For this review, take the finished solid that the model builds, in its own axes (mm). A direction names the side the tool comes from. Coordinates: 2 decimals unless noted, no trailing zeros. Order: outer loops, then holes, each group sorted by start corner. A loop starts at its lowest first (then second) coordinate and runs counter-clockwise, first axis right, second up.
from build123d import *

# Parameters (mm, degrees)
F1_DEPTH  = 8
F0_R      = 3.1
F0_R_2    = 1.375
F2_DEPTH  = 3
F3_DEPTH  = 8
F4_W      = 7.5
F4_H      = 5
F5_DEPTH  = 3
F4_W_2    = 15
F4_W_3    = 6
F6_DEPTH  = 3
F7_W      = 15.9
F7_H      = 5
F7_W_2    = 13.1
F8_DEPTH  = 3
F9_W      = 14.6
F9_H      = 5
F10_DEPTH = 3
F11_DEPTH = 10


with BuildPart() as f1:
    # F0 (on Top) → F1 (new body)
    with BuildSketch(Plane.XY):
        with BuildLine():
            Line((82, 59), (3, 59))
            ThreePointArc((3, 59), (-1.242641, 57.242641), (-3, 53))
            Line((-3, 53), (-3, 3))
            ThreePointArc((-3, 3), (-1.242641, -1.242641), (3, -3))
            Line((3, -3), (82, -3))
            ThreePointArc((82, -3), (86.242641, -1.242641), (88, 3))
            Line((88, 3), (88, 53))
            ThreePointArc((88, 53), (86.242641, 57.242641), (82, 59))
        make_face()
        with BuildLine():
            Line((82, 0), (3, 0))
            ThreePointArc((3, 0), (0.87868, 0.87868), (0, 3))
            Line((0, 3), (0, 53))
            ThreePointArc((0, 53), (0.87868, 55.12132), (3, 56))
            Line((3, 56), (82, 56))
            ThreePointArc((82, 56), (84.12132, 55.12132), (85, 53))
            Line((85, 53), (85, 3))
            ThreePointArc((85, 3), (84.12132, 0.87868), (82, 0))
        make_face(mode=Mode.SUBTRACT)
    extrude(amount=F1_DEPTH)

    # F0 (on Top) → F2 (join)
    with BuildSketch(Plane.XY):
        with BuildLine():
            Line((82, 59), (3, 59))
            ThreePointArc((3, 59), (-1.242641, 57.242641), (-3, 53))
            Line((-3, 53), (-3, 3))
            ThreePointArc((-3, 3), (-1.242641, -1.242641), (3, -3))
            Line((3, -3), (82, -3))
            ThreePointArc((82, -3), (86.242641, -1.242641), (88, 3))
            Line((88, 3), (88, 53))
            ThreePointArc((88, 53), (86.242641, 57.242641), (82, 59))
        make_face()
        with BuildLine():
            Line((82, 0), (3, 0))
            ThreePointArc((3, 0), (0.87868, 0.87868), (0, 3))
            Line((0, 3), (0, 53))
            ThreePointArc((0, 53), (0.87868, 55.12132), (3, 56))
            Line((3, 56), (82, 56))
            ThreePointArc((82, 56), (84.12132, 55.12132), (85, 53))
            Line((85, 53), (85, 3))
            ThreePointArc((85, 3), (84.12132, 0.87868), (82, 0))
        make_face(mode=Mode.SUBTRACT)
        with BuildLine():
            ThreePointArc((0, 3), (0.87868, 0.87868), (3, 0))
            Line((3, 0), (82, 0))
            ThreePointArc((82, 0), (84.12132, 0.87868), (85, 3))
            Line((85, 3), (85, 53))
            ThreePointArc((85, 53), (84.12132, 55.12132), (82, 56))
            Line((82, 56), (3, 56))
            ThreePointArc((3, 56), (0.87868, 55.12132), (0, 53))
            Line((0, 53), (0, 3))
        make_face()
        with Locations((3.5, 3.5)):
            Circle(F0_R, mode=Mode.SUBTRACT)
        with Locations((61.5, 3.5)):
            Circle(F0_R, mode=Mode.SUBTRACT)
        with Locations((3.5, 52.5)):
            Circle(F0_R, mode=Mode.SUBTRACT)
        with Locations((61.5, 52.5)):
            Circle(F0_R, mode=Mode.SUBTRACT)
        with Locations((3.5, 3.5)):
            Circle(F0_R)
        with Locations((3.5, 3.5)):
            Circle(F0_R_2, mode=Mode.SUBTRACT)
        with Locations((3.5, 3.5)):
            Circle(F0_R_2)
        with Locations((61.5, 3.5)):
            Circle(F0_R)
        with Locations((61.5, 3.5)):
            Circle(F0_R_2, mode=Mode.SUBTRACT)
        with Locations((61.5, 3.5)):
            Circle(F0_R_2)
        with Locations((61.5, 52.5)):
            Circle(F0_R)
        with Locations((61.5, 52.5)):
            Circle(F0_R_2, mode=Mode.SUBTRACT)
        with Locations((61.5, 52.5)):
            Circle(F0_R_2)
        with Locations((3.5, 52.5)):
            Circle(F0_R)
        with Locations((3.5, 52.5)):
            Circle(F0_R_2, mode=Mode.SUBTRACT)
        with Locations((3.5, 52.5)):
            Circle(F0_R_2)
    extrude(amount=F2_DEPTH)

    # F0 (on Top) → F3 (join)
    with BuildSketch(Plane.XY):
        with Locations((3.5, 3.5)):
            Circle(F0_R_2)
        with Locations((61.5, 3.5)):
            Circle(F0_R_2)
        with Locations((3.5, 52.5)):
            Circle(F0_R_2)
        with Locations((61.5, 52.5)):
            Circle(F0_R_2)
    extrude(amount=F3_DEPTH)

    # F4 (on face) → F5 (cut, through all)
    with BuildSketch(Plane.XZ.offset(3)):
        with Locations((10.6, 5.5)):
            Rectangle(F4_W, F4_H)
    extrude(amount=-F5_DEPTH, mode=Mode.SUBTRACT)

    # F4 (on face) → F6 (cut, through all)
    with BuildSketch(Plane.XZ.offset(3)):
        with Locations((10.6, 5.5)):
            Rectangle(F4_W, F4_H)
        with Locations((32, 5.5)):
            Rectangle(F4_W_2, F4_H)
        with Locations((53.5, 5.5)):
            Rectangle(F4_W_3, F4_H)
    extrude(amount=-F6_DEPTH, mode=Mode.SUBTRACT)

    # F7 (on face) → F8 (cut, through all)
    with BuildSketch(Plane.YZ.offset(88)):
        with Locations((10.25, 5.5)):
            Rectangle(F7_W, F7_H)
        with Locations((29, 5.5)):
            Rectangle(F7_W_2, F7_H)
        with Locations((47, 5.5)):
            Rectangle(F7_W_2, F7_H)
    extrude(amount=-F8_DEPTH, mode=Mode.SUBTRACT)

    # F9 (on face) → F10 (cut, through all)
    with BuildSketch(Plane(origin=(-3, 0, 0), x_dir=(0, -1, 0), z_dir=(-1, 0, 0))):
        with Locations((-28, 5.5)):
            Rectangle(F9_W, F9_H)
    extrude(amount=-F10_DEPTH, mode=Mode.SUBTRACT)

    # F7 (on face) → F11 (cut)
    with BuildSketch(Plane.YZ.offset(88)):
        with Locations((10.25, 5.5)):
            Rectangle(F7_W, F7_H)
        with Locations((29, 5.5)):
            Rectangle(F7_W_2, F7_H)
        with Locations((47, 5.5)):
            Rectangle(F7_W_2, F7_H)
    extrude(amount=-F11_DEPTH, mode=Mode.SUBTRACT)


solid = f1.part
1. Take a section at B-B, the plane x = 23. Give the boundary of the cut face in (y, z).
Answer below:
outline: (-3, 0) - (59, 0) - (59, 8) - (56, 8) - (56, 3) - (0, 3) - (0, 8) - (-3, 8) - close
2. Take a section at D-D, the plane x = 61.5. Give the boundary of the cut face in (y, z) (3 decimals).
Answer below:
outline: (-3, 0) - (59, 0) - (59, 8) - (56, 8) - (56, 3) - (53.875, 3) - (53.875, 8) - (51.125, 8) - (51.125, 3) - (4.875, 3) - (4.875, 8) - (2.125, 8) - (2.125, 3) - (0, 3) - (0, 8) - (-3, 8) - close
3. The part is to be moulded in two halves that separate along X. For faces 5 (the face through (-0.3, 6.4, 8)), 6 (the face through (85, 38, 5)), 7 (the face through (88, 28, 2)), 8 (the face through (24.5, -2, 5)), say which applies: +X half, -X half, draft (parallel to the pull), parting line (faces both ways), or undercut.
Answer below:
face 5: draft
face 6: undercut
face 7: +X half
face 8: undercut
4. Machinability: for faces 1 (the face through (-2, 20.7, 5)), 2 (the face through (87, 18.2, 5)), 3 (the face through (50.5, -2, 5)), 4 (the face through (19, 0, 5)), which of the approach directions +Z, -Z, +X, -X, +Y, -Y give a long, thin tool a straight path to every point of the face, cutting with its end or side? Answer none if there is none.
Answer below:
face 1: +Z, -X
face 2: +Z, +X
face 3: +Z, -Y
face 4: +Z
5. Take a section at A-A, the plane z = 4. Give the number of separate pieces and of enclosed holes in the cut face, plus the area to 3 significant figures.
Answer below:
separate pieces: 11
enclosed holes: 0
area: 627 mm2
6. To check wall thickness, follow L1, parallel to Y at x = 70.5, z = 5.5; L2, parallel to Y at x = 53, z = 7; L3, parallel to Z at x = 6, y = 7.5. State the ranges of each line that lie inside material, in increasing order.
Answer below:
L1: y = -3 to 0, 56 to 59
L2: y = 56 to 59
L3: z = 0 to 3
7. Take a section at C-C, the plane y = 6.5. Give the boundary of the cut face in (x, z).
Answer below:
outline: (-3, 0) - (88, 0) - (88, 3) - (0, 3) - (0, 8) - (-3, 8) - close
8. Clearance check with flat-ended pins moving along their axes: pin 1 Ø1.5 at (x, z) = (-1, 5.5) entering from -Y; pin 2 Ø1 at (x, y) = (10, 13) entering from +Z; pin 3 Ø3.5 at (y, z) = (-1.5, 5) entering from -X; pin 4 Ø4.5 at (y, z) = (21, 5.5) entering from -X. State where each tip first meets the part, or that it passes through.
Answer below:
pin 1: stops at y = -2.04
pin 2: stops at z = 3
pin 3: stops at x = -2.33
pin 4: stops at x = -3
